Geometry: final body of the model. Coordinates: model frame, mm. Give positions to 0.01 mm unless a question says otherwise; leave off trailing zeros. Order: outer loops, then holes, each group sorted by start corner. A loop starts at its lowest first (then second) coordinate and runs counter-clockwise, first axis right, second up. Notation, with made-up numbers: M -8.5,-20 L 50.5,-20 A11 ccw 50.5,-3 Z; hole C -17.5,-13.5 d1. An arc over 180 degrees is marked long. One line per item, written item: value. Start each with the question number.
```python
from build123d import *

# Parameters (mm, degrees)
SKETCH1_R           = 3.175
BOSS_EXTRUDE1_DEPTH = 5.5626
FILLET1_R           = 0.254
FILLET2_R           = 0.762


with BuildPart() as part:
    # Sketch1 → Boss-Extrude1 (new body)
    with BuildSketch(Plane.XY):
        Polygon((3.207902433, -5.55625), (6.415804866, 0), (3.207902433, 5.55625), (-3.207902433, 5.55625), (-6.415804866, 0), (-3.207902433, -5.55625), align=None)
        with Locations(Location((0, 0, 0), (0, 0, 180))):
            Circle(SKETCH1_R, mode=Mode.SUBTRACT)
    extrude(amount=BOSS_EXTRUDE1_DEPTH)

    # Fillet1
    fillet1_edges = [part.edges().sort_by_distance(p)[0] for p in [
        (-4.81185365, 2.778125, 5.5626),
        (6.415804866, 0, 2.7813),
        (3.207902433, -5.55625, 2.7813),
        (-3.207902433, -5.55625, 2.7813),
        (-6.415804866, 0, 2.7813),
        (-3.207902433, 5.55625, 2.7813),
        (3.207902433, 5.55625, 2.7813),
        (-4.81185365, -2.778125, 5.5626),
        (0, -5.55625, 5.5626),
        (4.81185365, -2.778125, 5.5626),
        (4.81185365, 2.778125, 5.5626),
        (4.81185365, -2.778125, 0),
        (0, -5.55625, 0),
        (-4.81185365, -2.778125, 0),
        (0, 5.55625, 5.5626),
        (-4.81185365, 2.778125, 0),
        (0, 5.55625, 0),
        (4.81185365, 2.778125, 0),
    ]]
    fillet(fillet1_edges, radius=FILLET1_R)

    # Fillet2
    fillet2_edges = [part.edges().sort_by_distance(p)[0] for p in [
        (3.175, 0, 0),
        (3.175, 0, 5.5626),
    ]]
    fillet(fillet2_edges, radius=FILLET2_R)


solid = part.part
```
Q1. Mould query, pull axis X, two halves, no side actions, for faces 1 (the face through (-1.5, 2.8, 2.8)), 2 (the face through (4, -1, 5.563)), 3 (the face through (-4.7, -2.8, 5.5)), 4 (the face through (4.77, -2.7, 5.49)). Classes: +X half, -X half, draft (parallel to the pull), parting line (faces both ways), or undercut.
Q2. Ray query, line 1 along Y through (x, z) = (0, 2.7) (3 decimals); line 2 along Z through (x, y) = (-0.25, -3.5); line 3 along X through (y, z) = (-0.5, 0.35). Return the intervals inside material, ascending. Write a range as [from, to].
Q3. Section query B-B on x = 0. Return loops of the section in (y, z) (3 decimals), and give its area (3 significant figures).
Q4. Section query A-A on z = 4.4. Return loops of the section in (x, y) (3 decimals), and give its area (3 significant figures).
Q5. Section query C-C on z = 0.5. Return loops of the section in (x, y).
Q6. Contact query for flat-ended pins moving along their axis: pin 1 (3 mm diameter, centred on y = 4, z = 2, fed in from -X); pin 2 (6 mm diameter, centred on x = -3.5, y = 0, fed in from -Z). Output: stop coordinate, or through.
Results below:
1. face 1: undercut
1. face 2: draft
1. face 3: -X half
1. face 4: +X half
2. line 1: [-5.556, -3.175], [3.175, 5.556]
2. line 2: [0.13, 5.43]
2. line 3: [-6.13, -3.26], [3.26, 6.13]
3. outline: M -5.556,0.254 A0.254 ccw -5.302,0 L -3.937,0 A0.762 ccw -3.175,0.762 L -3.175,4.801 A0.762 ccw -3.937,5.563 L -5.302,5.563 A0.254 ccw -5.556,5.309 Z; M 3.175,0.762 A0.762 ccw 3.937,0 L 5.302,0 A0.254 ccw 5.556,0.254 L 5.556,5.309 A0.254 ccw 5.302,5.563 L 3.937,5.563 A0.762 ccw 3.175,4.801 Z
3. area: 25.9 mm2
4. outline: M -6.342,-0.127 L -3.281,-5.429 A0.254 ccw -3.061,-5.556 L 3.061,-5.556 A0.254 ccw 3.281,-5.429 L 6.342,-0.127 A0.254 ccw 6.342,0.127 L 3.281,5.429 A0.254 ccw 3.061,5.556 L -3.061,5.556 A0.254 ccw -3.281,5.429 L -6.342,0.127 A0.254 ccw Z; hole C 0,0 d6.35
4. area: 75.3 mm2
5. outline: M -6.34,-0.13 L -3.28,-5.43 A0.25 ccw -3.06,-5.56 L 3.06,-5.56 A0.25 ccw 3.28,-5.43 L 6.34,-0.13 A0.25 ccw 6.34,0.13 L 3.28,5.43 A0.25 ccw 3.06,5.56 L -3.06,5.56 A0.25 ccw -3.28,5.43 L -6.34,0.13 A0.25 ccw Z; hole C 0,0 d6.44
6. pin 1: x = -4.97
6. pin 2: z = 0
